Geometry check sheet. Reference: the model listing, model coordinates, mm. A direction names the side the tool comes from. Coordinates: 2 decimals unless noted, no trailing zeros. Order: outer loops, then holes, each group sorted by start corner. A loop starts at its lowest first (then second) coordinate and runs counter-clockwise, first axis right, second up.
```python
from build123d import *

# Parameters (mm, degrees)
F0_W     = 203.2
F0_H     = 127
F1_DEPTH = 127
F3_DEPTH = 76.2
F4_SIZE2 = 101.6
F4_SIZE  = 76.2
F5_R     = 5.08
F6_R     = 15.24
F7_DEPTH = 50.8
F8_R     = 15.24
F9_DEPTH = 127


with BuildPart() as f1:
    # F0 (on Front) → F1 (new body)
    with BuildSketch(Plane.XZ):
        Rectangle(F0_W, F0_H)
    extrude(amount=F1_DEPTH)

    # F2 (on face) → F3 (cut)
    with BuildSketch(Plane.XZ.offset(127)):
        Polygon((-38.1, 0), (-38.1, -63.5), (101.6, -63.5), (101.6, 63.5), (0, 63.5), (0, 0), align=None)
    extrude(amount=-F3_DEPTH, mode=Mode.SUBTRACT)

    # F4
    f4_edges = [f1.edges().sort_by_distance(p)[0] for p in [
        (101.6, -25.4, 63.5),
    ]]
    f4_side = f1.faces().sort_by_distance((-21.771429, -52.614286, 63.5))[0]
    chamfer(f4_edges, length=F4_SIZE, length2=F4_SIZE2, reference=f4_side)

    # F5
    f5_edges = [f1.edges().sort_by_distance(p)[0] for p in [
        (-50.8, -127, 63.5),
        (-19.05, -127, 0),
        (0, -88.9, 63.5),
        (0, -88.9, 0),
        (12.7, -50.8, 63.5),
        (25.4, -25.4, 63.5),
        (-38.1, 0, 63.5),
        (-38.1, -88.9, -63.5),
        (-69.85, -127, -63.5),
        (-38.1, -127, -31.75),
        (-101.6, -127, 0),
        (31.75, -50.8, -63.5),
        (101.6, -25.4, -63.5),
        (-38.1, -50.8, -31.75),
        (0, -50.8, 31.75),
        (-38.1, -88.9, 0),
        (0, 0, -63.5),
        (-101.6, -63.5, -63.5),
        (-101.6, 0, 0),
        (-19.05, -50.8, 0),
    ]]
    fillet(f5_edges, radius=F5_R)

    # F6 (on face) → F7 (cut, through all)
    with BuildSketch(Plane.XZ.offset(50.8)):
        with Locations((17.78, -17.78)):
            Circle(F6_R)
    extrude(amount=-F7_DEPTH, mode=Mode.SUBTRACT)

    # F8 (on face) → F9 (cut, through all)
    with BuildSketch(Plane.XY.offset(63.5)):
        with Locations((-64.6355301142, -57.3951564729)):
            Circle(F8_R)
    extrude(amount=-F9_DEPTH, mode=Mode.SUBTRACT)


solid = f1.part
```
Item 1: Sectioned sample at D-D (z = 44). Record the cut outline in (x, y) (3 decimals).
Item 2: Sectioned sample at A-A (x = 17.78). Record the cut outline in (y, z).
Item 3: Thickness scan on line 1 along Z through (x, y) = (17, -40); line 2 along Z through (x, y) = (17.78, -39); line 3 along Y through (x, z) = (-65, -42.5). Record the ranges inside material, lowest first.
Item 4: Sectioned sample at C-C (y = -24). Record the cut outline in (x, z), and give its area (3 significant figures).
Item 5: Sectioned sample at B-B (z = -8). Record the cut outline in (x, y) (3 decimals), and give its area (3 significant figures).
Item 6: Tool access check on faces 1 (the face through (-16.741, -125.551, 1.528)), 2 (the face through (-40, -63, 63.5)), 3 (the face through (14.295, -49.272, 62.051)). Record the directions out of +Z, -Z, +X, -X, +Y, -Y that give a thin tool (end or side, any length) a straight path to the whole face; none if there is none.
Item 7: Depth check by flat-ended pin: P1, Ø2, axis at y = -85, z = 33.5, coming from the +X side; P2, Ø8.5, axis at x = -21, y = -76.5, coming from the -Z side; P3, Ø16, axis at y = -98.5, z = -43.5, coming from the +X side. Enter the tip coordinate at first touch or a pass-through.
Item 8: Release check for a two-part mould opening along Y. For faces 4 (the face through (-76.73, -66.67, 0.89)), 5 (the face through (-1.449, -90.942, 1.528)), 6 (the face through (1.528, -52.249, 31.377)), 7 (the face through (-21, 0, 1)) record: pulls with the +Y half, pulls with the -Y half, needs draft (parallel to the pull), parting line crosses it, or undercut.
Geometry check:
1. outline: (-101.6, -121.92) arc R5.08 ccw to (-96.52, -127) - (0, -127) - (0, -55.88) arc R5.08 cw to (5.08, -50.8) - (40.025, -50.8) - (40.025, 0) - (-96.52, 0) arc R5.08 ccw to (-101.6, -5.08) - close; hole circle Ø30.48 at (-64.636, -57.395)
2. outline: (-50.8, -58.42) arc R5.08 ccw to (-45.72, -63.5) - (-5.08, -63.5) arc R5.08 ccw to (0, -58.42) - (0, -33.02) - (-50.8, -33.02) - close; (-50.8, -2.54) - (0, -2.54) - (0, 58.42) arc R5.08 ccw to (-5.08, 63.5) - (-45.72, 63.5) arc R5.08 ccw to (-50.8, 58.42) - close
3. line 1: z = -63.5 to -33, -2.56 to 63.5
3. line 2: z = -63.5 to -33.02, -2.54 to 63.5
3. line 3: y = -127 to -72.63, -42.16 to 0
4. outline: (-101.6, -58.42) arc R5.08 ccw to (-96.52, -63.5) - (96.52, -63.5) arc R5.08 ccw to (101.6, -58.42) - (101.6, -38.1) - (26.92, 61.47) arc R5.08 ccw to (22.86, 63.5) - (-101.6, 63.5) - close; hole circle Ø30.48 at (17.78, -17.78)
4. area: 21,200 mm2
5. outline: (-101.6, -121.92) arc R5.08 ccw to (-96.52, -127) - (-43.18, -127) arc R5.08 ccw to (-38.1, -121.92) - (-38.1, -55.88) arc R5.08 cw to (-33.02, -50.8) - (6.092, -50.8) - (6.092, 0) - (-96.52, 0) arc R5.08 ccw to (-101.6, -5.08) - close; (29.468, -50.8) - (79.025, -50.8) - (79.025, 0) - (29.468, 0) - close; hole circle Ø30.48 at (-64.636, -57.395)
5. area: 12,100 mm2
6. face 1: -Z, +X, -Y
6. face 2: +Z, +X, -X, +Y, -Y
6. face 3: +Z, +X, -Y
7. P1: stops at x = 0
7. P2: stops at z = 0
7. P3: stops at x = -38.1
8. face 4: undercut
8. face 5: needs draft
8. face 6: pulls with the -Y half
8. face 7: pulls with the +Y half
